Geometry check sheet. Reference: drawing and pictorial views, mm from the part's lowest x, y, z. A direction names the side the tool comes from. Round coordinates to 2 decimals unless told otherwise and drop trailing zeros. Write each loop counter-clockwise with the first axis right and the second up, starting at its lowest first coordinate (ties: lowest second). Pieces come first, ordered by that corner, then holes.
Item 1: Section check D-D, the plane y = 29. Record the cut outline in (x, z).
Item 2: Depth check by flat-ended pin: pin 1 (6 mm diameter, centred on x = 14.5, z = 13, fed in from +Y); pin 2 (6 mm diameter, centred on y = 23, z = 11.5, fed in from -X); pin 3 (5 mm diameter, centred on y = 28, z = 9, fed in from +X). Enter the tip coordinate at first touch or a pass-through.
Item 3: Material ranges on line 1 along X through (y, z) = (37.85, 10); line 2 along Z through (x, y) = (45, 38); line 3 along X through (y, z) = (33.5, 6), recorded low to high.
Item 4: Set-up check for the marked faces 1, 2 and 3: record each of +Z, -Z, +X, -X, +Y, -Y from which the full face is reachable in a straight line by a thin tool's end or side.
Item 5: Section check A-A, the plane x = 45. Record the cut outline in (y, z).
Item 6: Section check B-B, the plane z = 10. Record the cut outline in (x, y), plus the area to 3 significant figures.
Item 7: Section check C-C, the plane z = 17.75. Record the cut outline in (x, y).
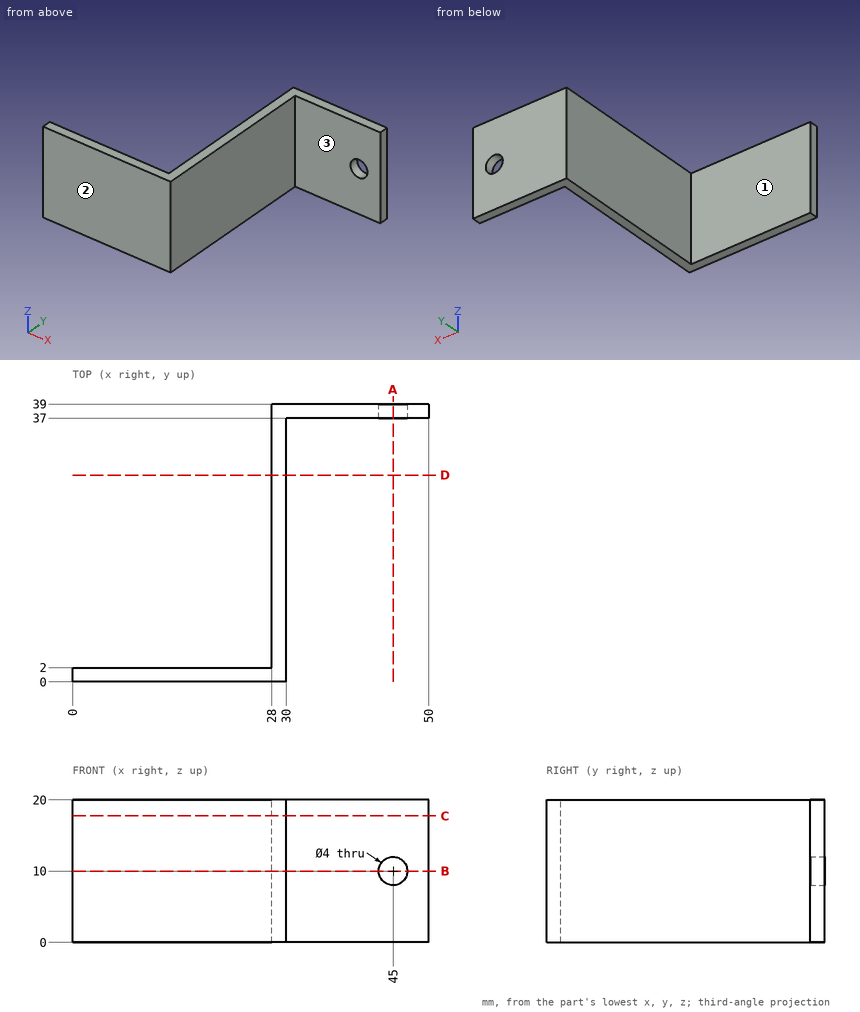
Values found:
1. outline: (28, 0) - (30, 0) - (30, 20) - (28, 20) - close
2. pin 1: stops at y = 2
2. pin 2: stops at x = 28
2. pin 3: stops at x = 30
3. line 1: x = 28 to 43, 47 to 50
3. line 2: z = 0 to 8, 12 to 20
3. line 3: x = 28 to 30
4. face 1: +Z, -Z, -X, +Y
4. face 2: +Z, -Z, +X, -X, -Y
4. face 3: +Z, -Z, +X, -Y
5. outline: (37, 0) - (39, 0) - (39, 8) - (37, 8) - close; (37, 12) - (39, 12) - (39, 20) - (37, 20) - close
6. outline: (0, 0) - (30, 0) - (30, 37) - (43, 37) - (43, 39) - (28, 39) - (28, 2) - (0, 2) - close; (47, 37) - (50, 37) - (50, 39) - (47, 39) - close
6. area: 166 mm2
7. outline: (0, 0) - (30, 0) - (30, 37) - (50, 37) - (50, 39) - (28, 39) - (28, 2) - (0, 2) - close
